Design review of the part built by this model. Coordinates are the model's own, in mm. A direction names the side the tool comes from. Give positions to 0.01 mm unless a question says otherwise; leave off trailing zeros. Loops run counter-clockwise (first coordinate to the right, second up) from the corner with the lowest first, then second, coordinate; pieces in that order, holes last. Notation, with made-up numbers: M 44.25,45.5 L 48.25,45.5 A31 ccw 48.25,70.5 Z; hole C 27,75.25 d10. An arc over 180 degrees is marked long. Use CSV: the item, a comma, the result in double quotes.
from build123d import *

# Parameters (mm, degrees)
F0_W     = 25.4
F0_H     = 63.5
F1_DEPTH = 6.35
F2_W     = 25.4
F2_H     = 6.35
F3_DEPTH = 82.55
F5_DEPTH = 25.4
F6_W     = 57.15
F6_H     = 6.35
F7_DEPTH = 25.4


with BuildPart() as f1:
    # F0 (on Top) → F1 (new body)
    with BuildSketch(Plane.XY):
        with Locations((4.9058877259, -6.6879848838)):
            Rectangle(F0_W, F0_H)
    extrude(amount=F1_DEPTH)

    # F2 (on face) → F3 (join)
    with BuildSketch(Plane(origin=(0, 0, 0), x_dir=(1, 0, 0), z_dir=(0, 0, -1))):
        with Locations((4.9058877259, -21.8870151162)):
            Rectangle(F2_W, F2_H)
    extrude(amount=F3_DEPTH)

    # F4 (on face) → F5 (cut)
    with BuildSketch(Plane(origin=(0, 25.0620151162, 0), x_dir=(-1, 0, 0), z_dir=(0, 1, 0))):
        with BuildLine():
            Line((-6.1758877259, -16.51), (-11.2558877259, -16.51))
            Line((-11.2558877259, -16.51), (-11.2558877259, -21.59))
            ThreePointArc((-11.2558877259, -21.59), (-7.6637852775, -20.1021024484), (-6.1758877259, -16.51))
        make_face()
        with BuildLine():
            Line((-11.2558877259, -21.59), (-11.2558877259, -16.51))
            Line((-11.2558877259, -16.51), (-16.3358877259, -16.51))
            ThreePointArc((-16.3358877259, -16.51), (-14.8479901744, -20.1021024484), (-11.2558877259, -21.59))
        make_face()
        with BuildLine():
            Line((-11.2558877259, -16.51), (-11.2558877259, -11.43))
            ThreePointArc((-11.2558877259, -11.43), (-14.8479901744, -12.9178975516), (-16.3358877259, -16.51))
            Line((-16.3358877259, -16.51), (-11.2558877259, -16.51))
        make_face()
        with BuildLine():
            Line((1.4441122717, -11.43), (-11.2558877259, -11.43))
            ThreePointArc((-11.2558877259, -11.43), (-7.6637852775, -12.9178975516), (-6.1758877259, -16.51))
            Line((-6.1758877259, -16.51), (-3.6358877259, -16.51))
            ThreePointArc((-3.6358877259, -16.51), (-2.1479901752, -12.9178975524), (1.4441122717, -11.43))
        make_face()
        with BuildLine():
            Line((1.4441122741, -16.51), (1.4441122741, -11.43))
            ThreePointArc((1.4441122717, -11.43), (-2.1479901752, -12.9178975524), (-3.6358877259, -16.51))
            Line((-3.6358877259, -16.51), (1.4441122741, -16.51))
        make_face()
        with BuildLine():
            ThreePointArc((6.5241122741, -16.51), (5.0362147216, -12.9178975507), (1.4441122717, -11.43))
            Line((1.4441122741, -11.43), (1.4441122741, -16.51))
            Line((1.4441122741, -16.51), (6.5241122741, -16.51))
        make_face()
        with BuildLine():
            Line((6.5241122741, -16.51), (1.4441122741, -16.51))
            Line((1.4441122741, -16.51), (1.4441122741, -21.59))
            ThreePointArc((1.4441122741, -21.59), (5.0362147225, -20.1021024484), (6.5241122741, -16.51))
        make_face()
        with BuildLine():
            Line((-3.6358877259, -16.51), (-6.1758877259, -16.51))
            ThreePointArc((-6.1758877259, -16.51), (-7.6637852775, -20.1021024484), (-11.2558877259, -21.59))
            Line((-11.2558877259, -21.59), (1.4441122741, -21.59))
            ThreePointArc((1.4441122741, -21.59), (-2.1479901744, -20.1021024484), (-3.6358877259, -16.51))
        make_face()
        with BuildLine():
            Line((1.4441122741, -21.59), (1.4441122741, -16.51))
            Line((1.4441122741, -16.51), (-3.6358877259, -16.51))
            ThreePointArc((-3.6358877259, -16.51), (-2.1479901744, -20.1021024484), (1.4441122741, -21.59))
        make_face()
        with BuildLine():
            ThreePointArc((-6.1758877259, -16.51), (-7.6637852775, -12.9178975516), (-11.2558877259, -11.43))
            Line((-11.2558877259, -11.43), (-11.2558877259, -16.51))
            Line((-11.2558877259, -16.51), (-6.1758877259, -16.51))
        make_face()
        with BuildLine():
            Line((-11.2558877259, -59.69), (-11.2558877259, -54.61))
            ThreePointArc((-11.2558877221, -54.61), (-14.847990173, -56.0978975502), (-16.3358877259, -59.69))
            Line((-16.3358877259, -59.69), (-11.2558877259, -59.69))
        make_face()
        with BuildLine():
            ThreePointArc((-6.1758877259, -59.69), (-7.6637852762, -56.0978975529), (-11.2558877221, -54.61))
            Line((-11.2558877259, -54.61), (-11.2558877259, -59.69))
            Line((-11.2558877259, -59.69), (-6.1758877259, -59.69))
        make_face()
        with BuildLine():
            Line((-6.1758877259, -59.69), (-11.2558877259, -59.69))
            Line((-11.2558877259, -59.69), (-11.2558877259, -64.77))
            ThreePointArc((-11.2558877259, -64.77), (-7.6637852775, -63.2821024484), (-6.1758877259, -59.69))
        make_face()
        with BuildLine():
            Line((-11.2558877259, -64.77), (-11.2558877259, -59.69))
            Line((-11.2558877259, -59.69), (-16.3358877259, -59.69))
            ThreePointArc((-16.3358877259, -59.69), (-14.8479901744, -63.2821024484), (-11.2558877259, -64.77))
        make_face()
        with BuildLine():
            Line((1.4441122741, -54.61), (-11.2558877221, -54.61))
            ThreePointArc((-11.2558877221, -54.61), (-7.6637852762, -56.0978975529), (-6.1758877259, -59.69))
            Line((-6.1758877259, -59.69), (-3.6358877259, -59.69))
            ThreePointArc((-3.6358877259, -59.69), (-2.1479901744, -56.0978975516), (1.4441122741, -54.61))
        make_face()
        with BuildLine():
            Line((1.4441122741, -59.69), (1.4441122741, -54.61))
            ThreePointArc((1.4441122741, -54.61), (-2.1479901744, -56.0978975516), (-3.6358877259, -59.69))
            Line((-3.6358877259, -59.69), (1.4441122741, -59.69))
        make_face()
        with BuildLine():
            Line((1.4441122741, -64.77), (1.4441122741, -59.69))
            Line((1.4441122741, -59.69), (-3.6358877259, -59.69))
            ThreePointArc((-3.6358877259, -59.69), (-2.1479901744, -63.2821024484), (1.4441122741, -64.77))
        make_face()
        with BuildLine():
            Line((-3.6358877259, -59.69), (-6.1758877259, -59.69))
            ThreePointArc((-6.1758877259, -59.69), (-7.6637852775, -63.2821024484), (-11.2558877259, -64.77))
            Line((-11.2558877259, -64.77), (1.4441122741, -64.77))
            ThreePointArc((1.4441122741, -64.77), (-2.1479901744, -63.2821024484), (-3.6358877259, -59.69))
        make_face()
        with BuildLine():
            ThreePointArc((6.5241122741, -59.69), (5.0362147225, -56.0978975516), (1.4441122741, -54.61))
            Line((1.4441122741, -54.61), (1.4441122741, -59.69))
            Line((1.4441122741, -59.69), (6.5241122741, -59.69))
        make_face()
        with BuildLine():
            Line((6.5241122741, -59.69), (1.4441122741, -59.69))
            Line((1.4441122741, -59.69), (1.4441122741, -64.77))
            ThreePointArc((1.4441122741, -64.77), (5.0362147225, -63.2821024484), (6.5241122741, -59.69))
        make_face()
    extrude(amount=-F5_DEPTH, mode=Mode.SUBTRACT)

    # F6 (on face) → F7 (cut)
    with BuildSketch(Plane(origin=(-7.7941122741, 0, 0), x_dir=(0, -1, 0), z_dir=(-1, 0, 0))):
        with Locations((9.8629848838, 3.175)):
            Rectangle(F6_W, F6_H)
    extrude(amount=-F7_DEPTH, mode=Mode.SUBTRACT)


solid = f1.part
(1) We need section A-A on x = 6.5. State the section outline as (y, z) points, then the cut area to 3 significant figures.
A:
outline,"M 18.71,-82.55 L 25.06,-82.55 L 25.06,-64.77 L 18.71,-64.77 Z; M 18.71,-54.61 L 25.06,-54.61 L 25.06,-21.59 L 18.71,-21.59 Z; M 18.71,-11.43 L 25.06,-11.43 L 25.06,6.35 L 18.71,6.35 Z"
area,"435 mm²"
(2) We need section C-C on x = 14.25. State the section outline as (y, z) points.
A:
outline,"M 18.71,-82.55 L 25.06,-82.55 L 25.06,-63.79 L 18.71,-63.79 Z; M 18.71,-55.59 L 25.06,-55.59 L 25.06,-20.61 L 18.71,-20.61 Z; M 18.71,-12.41 L 25.06,-12.41 L 25.06,6.35 L 18.71,6.35 Z"
(3) We need section B-B on y = 20.5. State the section outline as (x, z) points, then the cut area to 3 significant figures.
A:
outline,"M -7.79,-82.55 L 17.61,-82.55 L 17.61,6.35 L -7.79,6.35 Z; hole M -1.44,-64.77 L 11.26,-64.77 A5.08 ccw 11.26,-54.61 L -1.44,-54.61 A5.08 ccw Z; hole M -1.44,-21.59 L 11.26,-21.59 A5.08 ccw 11.26,-11.43 L -1.44,-11.43 A5.08 ccw Z"
area,"1,840 mm²"
(4) Wall thickness on line 1 along Z through (x, y) = (10.5, 20.75); line 2 along Z through (x, y) = (13.5, 23.25); line 3 along X through (y, z) = (23.5, -58): over which ranges is each line inside the solid? List them lowest first. Write a range as [from, to].
A:
line 1,"[-82.55, -64.77], [-54.61, -21.59], [-11.43, 6.35]"
line 2,"[-82.55, -64.25], [-55.13, -21.07], [-11.95, 6.35]"
line 3,"[-7.79, -6.23], [16.05, 17.61]"
(5) The part is to be moulded in two halves that separate along X. For faces 1 (the flat face through (5, 22, -64.77)), 2 (the flat face through (5, 22, -54.61)), 3 (the flat face through (-7.794, 22, -37)), 4 (the flat face through (5, 22, 6.35)), say which applies: released by +X, released by -X, zero draft, split by the parting line, or undercut.
A:
face 1,"undercut"
face 2,"undercut"
face 3,"released by -X"
face 4,"zero draft"
(6) Machinability: for faces 5 (the flat face through (5, 22, -21.59)), 6 (the flat face through (17.606, 22, -37)), which of the approach directions +Z, -Z, +X, -X, +Y, -Y give a long, thin tool a straight path to every point of the face, cutting with its end or side? Answer none if there is none.
A:
face 5,"+Y, -Y"
face 6,"+Z, -Z, +X, +Y, -Y"
